For this review, take the finished solid that the model builds, in its own axes (mm). Give positions to 0.01 mm unless a question says otherwise; leave off trailing zeros. Write each loop counter-clockwise with the first axis right and the second up, starting at its lowest first coordinate (ties: lowest second). Pieces come first, ordered by that corner, then holes. Notation, with made-up numbers: M -21,58.25 L -2,58.25 A23 ccw -2,91.25 Z; hole C 62,-26 d1. An arc over 180 degrees is marked long. Use one line per item in the form item = value. Start each with the question number.
Q1. Mouldability with a two-part tool opening along Y and no side actions: class faces 1 (the flat face through (-47.569, -17.03, -52.294)), 2 (the flat face through (-34, -34.544, -38)), 3 (the flat face through (-47.569, -2.504, -37.671)) as released by +Y, released by -Y, zero draft, split by the parting line, or undercut.
Q2. Consider section C-C on x = -48. Write out the cut boundary in (y, z), and give its area (3 significant figures).
Q3. Clearance check with a flat-ended pin moving along its axis: pin 1 Ø1 at (x, z) = (-46.5, -32) entering from +Y. State where the tip first meets the part, or that it passes through.
Q4. Consider section B-B on z = -47. Write out the cut boundary in (x, y).
Q5. For probe 1 along X at (y, z) = (-31, -32); probe 2 along Z at (x, y) = (-47, -27); probe 3 along X at (y, z) = (-30.5, -50), list the stretches that pass through material, from the lowest coordinate up. Write a range as [from, to].
Q6. Consider section A-A on y = -22.5. Write out the cut boundary in (x, z), and give its area (3 significant figures).
```python
from build123d import *

# Parameters (mm, degrees)
F1_E0_BOTTOM_W = 27.100160718
F1_E0_BOTTOM_H = 34.544
F2_DEPTH       = 33.782
F3_SIZE        = 5.08


with BuildPart() as f2:
    # F1_E0_bottom (on explicit) → F2 (new body)
    with BuildSketch(Plane(origin=(-50.1445159316, 0, -21.0164524615), x_dir=(1, 0, 0), z_dir=(0, 0, -1))):
        with Locations((13.550080359, 17.272)):
            Rectangle(F1_E0_BOTTOM_W, F1_E0_BOTTOM_H)
    extrude(amount=F2_DEPTH)

    # F3
    f3_edges = [f2.edges().sort_by_distance(p)[0] for p in [
        (-50.144516, -34.544, -37.907452),
        (-50.144516, 0, -37.907452),
        (-50.144516, -17.272, -21.016452),
        (-50.144516, -17.272, -54.798452),
    ]]
    chamfer(f3_edges, length=F3_SIZE)


solid = f2.part
```
Working result:
q1.face_1 = zero draft
q1.face_2 = released by -Y
q1.face_3 = released by +Y
q2.outline = M -31.61,-51.86 L -2.94,-51.86 L -2.94,-23.95 L -31.61,-23.95 Z
q2.area = 800 mm²
q3.pin_1 = -0.94
q4.outline = M -50.14,-29.46 L -45.06,-34.54 L -23.04,-34.54 L -23.04,0 L -45.06,0 L -50.14,-5.08 Z
q5.probe_1 = [-48.61, -23.04]
q5.probe_2 = [-52.86, -22.95]
q5.probe_3 = [-49.11, -23.04]
q6.outline = M -50.14,-49.72 L -45.06,-54.8 L -23.04,-54.8 L -23.04,-21.02 L -45.06,-21.02 L -50.14,-26.1 Z
q6.area = 890 mm²
